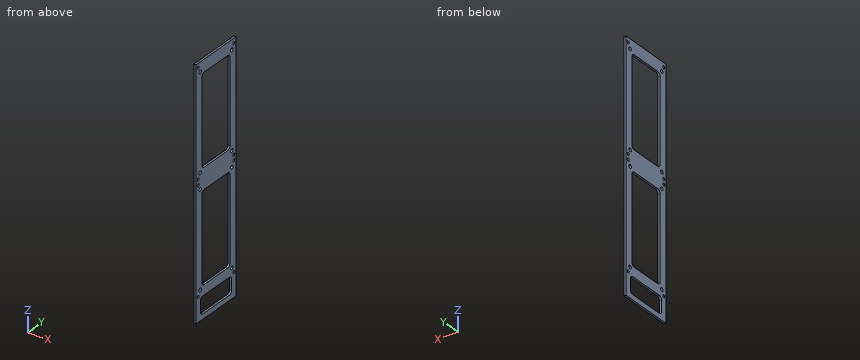
```python
from build123d import *

# Parameters (mm, degrees)
SKETCH1_W            = 390
SKETCH1_H            = 90
BOSS_EXTRUDE1_DEPTH  = 3.175
SKETCH2_W            = 143
SKETCH2_H            = 63
CUT_EXTRUDE1_DEPTH   = 3.175
M5_CLEARANCE_HOLE1_D = 5.5
SKETCH6_W            = 27
SKETCH6_H            = 70
CUT_EXTRUDE2_DEPTH   = 3.175
M4_CLEARANCE_HOLE2_D = 4.5
FILLET1_R            = 5


with BuildPart() as part:
    # Sketch1 → Boss-Extrude1 (new body)
    with BuildSketch(Plane(origin=(0, 0, 0), x_dir=(0, 0, -1), z_dir=(1, 0, 0))):
        Rectangle(SKETCH1_W, SKETCH1_H)
    extrude(amount=BOSS_EXTRUDE1_DEPTH)

    # Sketch2 → Cut-Extrude1 (cut)
    with BuildSketch(Plane(origin=(3.175, 0, 0), x_dir=(0, 0, -1), z_dir=(1, 0, 0))):
        with Locations((72.675, 0)):
            Rectangle(SKETCH2_W, SKETCH2_H)
        with Locations((-103.825, 0)):
            Rectangle(SKETCH2_W, SKETCH2_H)
    extrude(amount=-CUT_EXTRUDE1_DEPTH, mode=Mode.SUBTRACT)

    # M5 Clearance Hole1 (through all)
    with Locations(Plane(origin=(3.175, 0, 0), x_dir=(0, 0, -1), z_dir=(1, 0, 0))):
        with Locations((-103.825, 0), (-28.075, 35.75), (-179.575, -35.75), (-179.575, 35.75), (-28.075, -35.75), (72.675, 0), (148.425, 35.75), (-3.075, -35.75), (-3.075, 35.75), (148.425, -35.75)):
            Hole(M5_CLEARANCE_HOLE1_D / 2)

    # Sketch6 → Cut-Extrude2 (cut)
    with BuildSketch(Plane(origin=(3.175, 0, 0), x_dir=(0, 0, -1), z_dir=(1, 0, 0))):
        with Locations((173.5, 0)):
            Rectangle(SKETCH6_W, SKETCH6_H)
    extrude(amount=-CUT_EXTRUDE2_DEPTH, mode=Mode.SUBTRACT)

    # M4 Clearance Hole2 (through all)
    with Locations(Plane(origin=(3.175, 0, 0), x_dir=(0, 0, -1), z_dir=(1, 0, 0))):
        with Locations((-103.825, 0), (-19.825, 40), (-187.825, -40), (-187.825, 40), (-19.825, -40), (72.675, 0), (156.675, 40), (-11.325, -40), (-11.325, 40), (156.675, -40)):
            Hole(M4_CLEARANCE_HOLE2_D / 2)

    # Fillet1
    fillet1_edges = [part.edges().sort_by_distance(p)[0] for p in [
        (1.5875, 35, -187),
        (1.5875, -35, -187),
        (1.5875, -35, -160),
        (1.5875, 35, -160),
        (1.5875, 31.5, 32.325),
        (1.5875, -31.5, 32.325),
        (1.5875, -31.5, 175.325),
        (1.5875, 31.5, 175.325),
        (1.5875, 31.5, -144.175),
        (1.5875, -31.5, -144.175),
        (1.5875, -31.5, -1.175),
        (1.5875, 31.5, -1.175),
    ]]
    fillet(fillet1_edges, radius=FILLET1_R)


solid = part.part
```
Here's how the part is built. I have some questions about the finished solid (model axes, mm). Round coordinates to 2 decimals unless told otherwise and drop trailing zeros. Order: outer loops, then holes, each group sorted by start corner. A loop starts at its lowest first (then second) coordinate and runs counter-clockwise, first axis right, second up. Notation, with made-up numbers: M -33,-19.75 L -9,-19.75 A17 ccw -9,-7.75 Z; hole C 44.5,-14.75 d6. An arc over 180 degrees is marked long. Answer as CSV lines item,"result".
Item 1: Imagine slicing it at C-C on x = 0.75. Give the number of separate pieces and of enclosed holes in the cut face, and give its area (3 significant figures).
From the geometry:
separate pieces,"1"
enclosed holes,"19"
area,"14,900 mm2"
Item 2: Please list where these lines run through material, in increasing order: L1, parallel to Z at x = 2, y = 25 (3 decimals); L2, parallel to Z at x = 3.05, y = -27; L3, parallel to Y at x = 1.35, z = 99.5. Write a range as [from, to].
From the geometry:
L1,"[-195, -187], [-160, -144.175], [-1.175, 32.325], [175.325, 195]"
L2,"[-195, -187], [-160, -144.15], [-1.2, 32.35], [175.3, 195]"
L3,"[-45, -31.5], [31.5, 45]"
Item 3: Imagine slicing it at A-A on y = 21.5. List the corners of the cut face in (x, z) for me (3 decimals).
From the geometry:
outline,"M 0,-195 L 3.175,-195 L 3.175,-187 L 0,-187 Z; M 0,-160 L 3.175,-160 L 3.175,-144.175 L 0,-144.175 Z; M 0,-1.175 L 3.175,-1.175 L 3.175,32.325 L 0,32.325 Z; M 0,175.325 L 3.175,175.325 L 3.175,195 L 0,195 Z"
Item 4: Imagine slicing it at B-B on z = -122. List the corners of the cut face in (x, y) for me (3 decimals), and give its area (3 significant figures).
From the geometry:
outline,"M 0,-45 L 3.175,-45 L 3.175,-31.5 L 0,-31.5 Z; M 0,31.5 L 3.175,31.5 L 3.175,45 L 0,45 Z"
area,"85.7 mm2"
